Could you check a few things on this drawing? It's one solid part, dimensions in mm from its lowest x, y, z. A direction names the side the tool comes from. Coordinates: 2 decimals unless noted, no trailing zeros. Write each loop counter-clockwise with the first axis right and the second up, starting at its lowest first coordinate (ties: lowest second). Pieces come first, ordered by that corner, then holes.
Item 1: I want a section at B-B (x = 176.5). Please give me the cut outline in (y, z).
Item 2: Please list where these lines run through material, in increasing order: line 1 (Y direction, x = 165, z = 63.5); line 2 (X direction, y = 85, z = 82.5); line 3 (X direction, y = 89, z = 68).
Item 3: I want a section at C-C (x = 65.5). Please give me the cut outline in (y, z), and give its area (3 significant figures).
Item 4: I want a section at A-A (z = 50). Please give me the cut outline in (x, y) (1 decimal), and give its area (3 significant figures).
Item 5: I'm going to push flat-ended pins straight in: P1, Ø1, axis at x = 52, z = 55, coming from the +Y side; P2, Ø1, axis at x = 111.5, z = 14, coming from the -Y side; P3, Ø1.5, axis at x = 262, z = 47.5, coming from the +Y side. Where does each tip first touch, or does it pass through?
Item 6: I want a section at D-D (y = 129.5). Please give me the cut outline in (x, z).
Item 7: If we mould it in two halves opening along Y, with no side actions, what happens to the marked faces 1, 2 and 3? For each: pulls with the +Y half, pulls with the -Y half, needs draft (parallel to the pull), parting line crosses it, or undercut.
Item 8: For the marked faces 4, 5 and 6, which set-ups out of +Z, -Z, +X, -X, +Y, -Y let a thin tool reach every point of the face, with its end or its side?
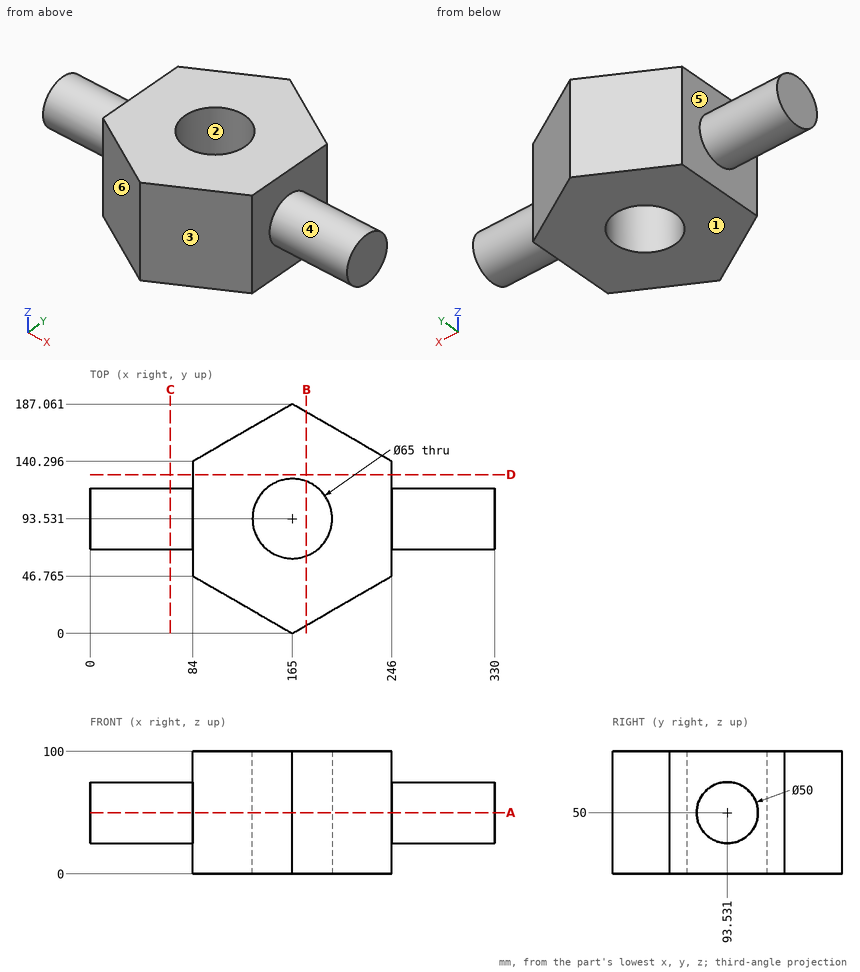
Answer:
1. outline: (6.64, 0) - (63.13, 0) - (63.13, 100) - (6.64, 100) - close; (123.93, 0) - (180.42, 0) - (180.42, 100) - (123.93, 100) - close
2. line 1: y = 0 to 61.03, 126.03 to 187.06
2. line 2: x = 84 to 133.64, 196.36 to 246
2. line 3: x = 0 to 132.82, 197.18 to 330
3. outline: circle Ø50 at (93.53, 50)
3. area: 1,960 mm2
4. outline: (0, 68.5) - (84, 68.5) - (84, 46.8) - (165, 0) - (246, 46.8) - (246, 68.5) - (330, 68.5) - (330, 118.5) - (246, 118.5) - (246, 140.3) - (165, 187.1) - (84, 140.3) - (84, 118.5) - (0, 118.5) - close; hole circle Ø65 at (165, 93.5)
4. area: 27,800 mm2
5. P1: stops at y = 118.12
5. P2: stops at y = 30.6
5. P3: stops at y = 118.47
6. outline: (84, 0) - (246, 0) - (246, 100) - (84, 100) - close
7. face 1: needs draft
7. face 2: undercut
7. face 3: pulls with the -Y half
8. face 4: +X
8. face 5: -X
8. face 6: +Z, -Z, -X, -Y
